For this review, use the dimensioned drawing (mm, ordinates from the lowest corner) and the shaded views. Round coordinates to 2 decimals unless told otherwise and drop trailing zeros. Loops run counter-clockwise (first coordinate to the right, second up) from the corner with the lowest first, then second, coordinate; pieces in that order, holes last. Notation, with made-up numbers: (1, -24) -> (38, -24) arc R12 cw to (38, -4) -> close; hole circle Ø9 at (-40, 20). An arc over 180 degrees is marked (long way). Answer as CSV lines item,"result". Start each with the question number.
(1) Take a section at B-B, the plane x = 82.55. Write out the cut boundary in (y, z) (3 decimals), and give its area (3 significant figures).
(2) Take a section at A-A, the plane y = 158.75. Write out the cut boundary in (x, z) (3 decimals).
(3) To check wall thickness, follow line 1 (Y direction, x = 19.05, z = 0.7) (3 decimals); line 2 (X direction, y = 262.89, z = 0.9) (3 decimals); line 3 (X direction, y = 158.75, z = 1) (3 decimals). State the ranges of each line that lie inside material, in increasing order. Write a range as from..to.
(4) Take a section at C-C, the plane y = 285.75. Write out the cut boundary in (x, z) (3 decimals), and give its area (3 significant figures).
(5) Draft analysis for pull direction Z (two halves, no side actions). For the marked faces 1 and 2, state which applies: +Z half, -Z half, draft (parallel to the pull), parting line (faces both ways), or undercut.
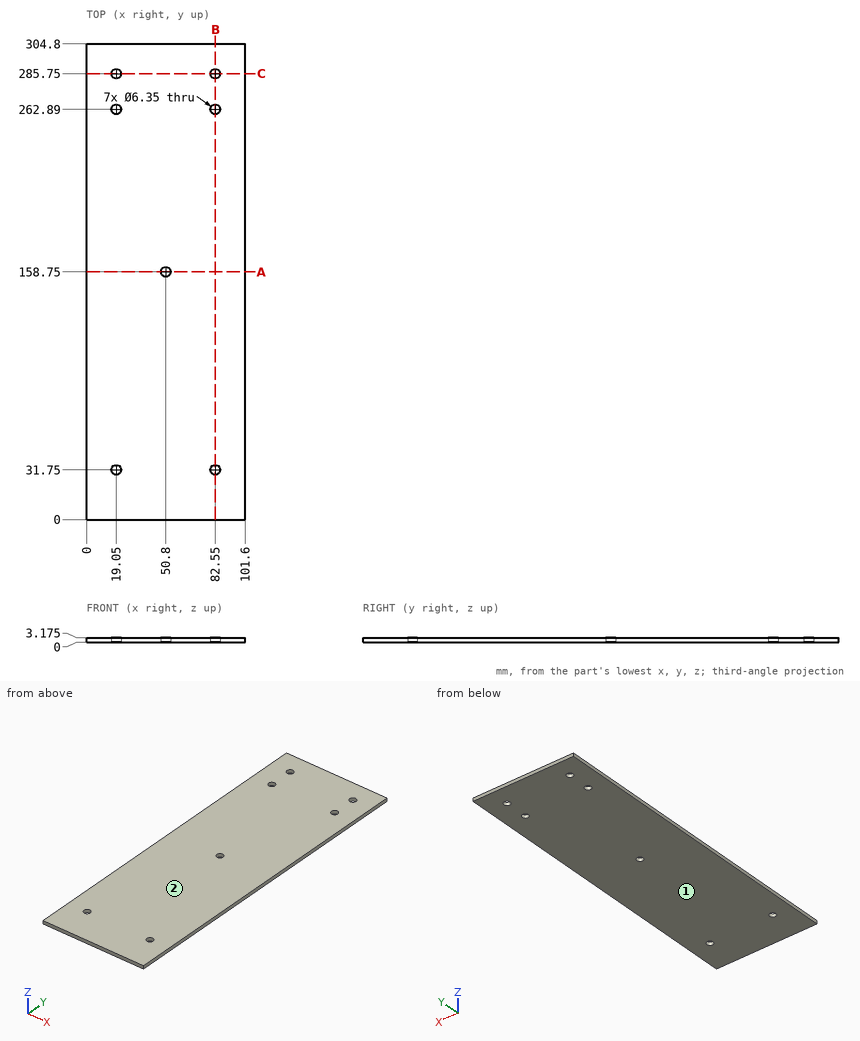
The answers:
1,outline,"(0, 0) -> (28.575, 0) -> (28.575, 3.175) -> (0, 3.175) -> close; (34.925, 0) -> (259.715, 0) -> (259.715, 3.175) -> (34.925, 3.175) -> close; (266.065, 0) -> (282.575, 0) -> (282.575, 3.175) -> (266.065, 3.175) -> close; (288.925, 0) -> (304.8, 0) -> (304.8, 3.175) -> (288.925, 3.175) -> close"
1,area,"907 mm²"
2,outline,"(0, 0) -> (47.625, 0) -> (47.625, 3.175) -> (0, 3.175) -> close; (53.975, 0) -> (101.6, 0) -> (101.6, 3.175) -> (53.975, 3.175) -> close"
3,line 1,"0..28.575, 34.925..259.715, 266.065..282.575, 288.925..304.8"
3,line 2,"0..15.875, 22.225..79.375, 85.725..101.6"
3,line 3,"0..47.625, 53.975..101.6"
4,outline,"(0, 0) -> (15.875, 0) -> (15.875, 3.175) -> (0, 3.175) -> close; (22.225, 0) -> (79.375, 0) -> (79.375, 3.175) -> (22.225, 3.175) -> close; (85.725, 0) -> (101.6, 0) -> (101.6, 3.175) -> (85.725, 3.175) -> close"
4,area,"282 mm²"
5,face 1,"-Z half"
5,face 2,"+Z half"
